Could you check a few things on this model? Use its own coordinates, in mm. Face numbers are marked on the shaded views. A direction names the side the tool comes from. Coordinates: 2 decimals unless noted, no trailing zeros. Loops run counter-clockwise (first coordinate to the right, second up) from the corner with the lowest first, then second, coordinate; pieces in that order, holes last. Notation, with made-up numbers: (45.5, -24.75) -> (79.5, -24.75) arc R17 ccw to (79.5, -3.75) -> close; hole circle Ø4 at (19, -26.75). An arc over 180 degrees is marked (long way). One line per question, with ' | ' between items. Start each with the question number.
(1) Which directions (+Z, -Z, +X, -X, +Y, -Y) give clear straight access to the entire face, cutting with the end or side of a thin tool? Please do the marked faces 4, 5 and 6.
(2) I'm going to push flat-ended pins straight in: pin 1 Ø3 at (x, y) = (63.41, -68.5) entering from -Z; pin 2 Ø8 at (x, y) = (-31, 20.5) entering from -Z; pin 3 Ø6 at (x, z) = (98.5, 6) entering from +Y; pin 4 Ø4 at (y, z) = (-39.5, -7.5) entering from +X. Where does each tip first touch, or does it pass through?
(3) If I drill on line 1 along Z through (x, y) = (46, 53.5); line 2 along X through (y, z) = (-3, 16); line 3 along Z through (x, y) = (-32, -21.5), over which ranges is the centre line in solid material (lowest first)?
(4) Suppose I cut it at A-A (x = -6.5). Please give me the cut outline in (y, z), plus the area to 3 significant figures.
(5) Suppose I cut it at B-B (x = -50). Please give me the cut outline in (y, z).
(6) If we mould it in two halves opening along X, with no side actions, what happens to the marked faces 1, 2 and 3? For each: pulls with the +X half, pulls with the -X half, needs draft (parallel to the pull), parting line crosses it, or undercut.
```python
from build123d import *

# Parameters (mm, degrees)
SKETCH1_4_RX        = 3.738629792
SKETCH1_4_RY        = 2.663157663
SKETCH1_4_R         = 0.723268125
SKETCH1_4_R_2       = 0.681301536
SKETCH1_4_R_3       = 0.980026241
SKETCH1_4_R_4       = 0.97959392
BOSS_EXTRUDE1_DEPTH = 0.254
BOSS_EXTRUDE2_DEPTH = 1.27
CIRPATTERN1_COUNT   = 4
FILLET1_R           = 1.27
SCALE1_SCALE        = 2.276
SKETCH2_R           = 2.38125
CUT_EXTRUDE1_DEPTH  = 50.083123014


with BuildPart() as part:
    # Sketch1 → Revolve1 (revolve)
    with BuildSketch(Plane.XY):
        with BuildLine():
            add(Edge.make_bspline(
                [(77.770736546, 14.197719485), (83.967767677, 14.197719485), (96.645248899, 10.827489794)],
                knots=[0, 0, 0, 1, 1, 1], degree=2))
            Line((96.645248899, 10.827489794), (96.645248899, 0))
            Line((96.645248899, 0), (17.093728294, 0))
            Line((17.093728294, 0), (17.093728294, 18.913287876))
            ThreePointArc((17.093728294, 18.913287876), (17.697865454, 20.511952721), (19.208297022, 21.311519777))
            Line((19.208297022, 21.311519777), (33.085444719, 21.311519777))
            Line((33.085444719, 21.311519777), (34.249634962, 20.65957324))
            Line((34.249634962, 20.65957324), (37.67078875, 20.65957324))
            Line((37.67078875, 20.65957324), (37.67078875, 21.107528589))
            Line((37.67078875, 21.107528589), (59.2694473, 21.107528589))
            Line((59.2694473, 21.107528589), (60.005153989, 20.695532843))
            Line((60.005153989, 20.695532843), (69.857537365, 20.695532843))
            Line((69.857537365, 20.695532843), (74.312442602, 17.349227048))
            Line((74.312442602, 17.349227048), (74.909379663, 17.349227048))
            Line((74.909379663, 17.349227048), (74.981675377, 14.952840317))
            Line((74.981675377, 14.952840317), (77.770736546, 14.952840317))
            Line((77.770736546, 14.952840317), (77.770736546, 14.197719485))
        make_face()
        with BuildLine():
            ThreePointArc((0, 0), (0.275579454, 2.642942048), (1.090462068, 5.172181663))
            Line((1.090462068, 5.172181663), (9.450406563, 5.172181663))
            Line((9.450406563, 5.172181663), (9.450406563, 0))
            Line((9.450406563, 0), (0, 0))
        make_face()
        Polygon((37.67078875, 18.679077388), (37.67078875, 20.65957324), (37.67078875, 21.107528589), (59.2694473, 21.107528589), (59.2694473, 18.679077388), align=None)
    revolve(axis=Axis((-26.796271974, 0, 0), (1, 0, 0)))

    # Sketch1_4 → Boss-Extrude1 (add, symmetric)
    with BuildSketch(Plane.XY):
        with BuildLine():
            ThreePointArc((57.062667076, 33.029408208), (58.562948924, 32.411407764), (59.192673253, 30.916009008))
            Line((59.192673253, 30.916009008), (59.2694473, 21.107528589))
            Line((59.2694473, 21.107528589), (37.67078875, 21.107528589))
            Line((37.67078875, 21.107528589), (37.67078875, 30.916009008))
            ThreePointArc((37.67078875, 30.916009008), (38.289789045, 32.410407913), (39.784187951, 33.029408208))
            Line((39.784187951, 33.029408208), (57.062667076, 33.029408208))
        make_face()
        with Locations((48.297023122, 27.463003731)):
            Ellipse(SKETCH1_4_RX, SKETCH1_4_RY, mode=Mode.SUBTRACT)
        with Locations((54.025364363, 23.762393902)):
            Circle(SKETCH1_4_R, mode=Mode.SUBTRACT)
        with Locations((42.682741772, 23.762393902)):
            Circle(SKETCH1_4_R_2, mode=Mode.SUBTRACT)
        with Locations((40.895803465, 30.126161394)):
            Circle(SKETCH1_4_R_3, mode=Mode.SUBTRACT)
        with Locations((55.916505535, 30.126161394)):
            Circle(SKETCH1_4_R_4, mode=Mode.SUBTRACT)
        Polygon((37.67078875, 18.679077388), (37.67078875, 20.65957324), (37.67078875, 21.107528589), (59.2694473, 21.107528589), (59.2694473, 18.679077388), align=None)
    boss_extrude1 = extrude(amount=BOSS_EXTRUDE1_DEPTH, both=True)

    # Sketch1_5 → Boss-Extrude2 (add, symmetric)
    with BuildSketch(Plane.XY):
        with BuildLine():
            ThreePointArc((11.014724068, 6.119928269), (10.364916389, 5.427600899), (9.450406563, 5.172181663))
            Line((9.450406563, 5.172181663), (9.450406563, 0))
            Line((9.450406563, 0), (12.123394722, 0))
            Line((12.123394722, 0), (12.123394722, 4.941548024))
            Line((12.123394722, 4.941548024), (17.093728294, 14.456770177))
            Line((17.093728294, 14.456770177), (17.093728294, 17.757592992))
            Line((17.093728294, 17.757592992), (11.971268091, 7.951139141))
            Line((11.971268091, 7.951139141), (11.014724068, 6.119928269))
        make_face()
    boss_extrude2 = extrude(amount=BOSS_EXTRUDE2_DEPTH, both=True)

    # Sketch1_6 → Cut-Revolve1 (revolve, cut)
    with BuildSketch(Plane.XY):
        with BuildLine():
            Line((9.450406563, 7.951139141), (9.450406563, 5.172181663))
            ThreePointArc((9.450406563, 5.172181663), (10.364916389, 5.427600899), (11.014724068, 6.119928269))
            Line((11.014724068, 6.119928269), (11.971268091, 7.951139141))
            Line((11.971268091, 7.951139141), (9.450406563, 7.951139141))
        make_face()
    cut_revolve1 = revolve(axis=Axis((-26.796271974, 0, 0), (1, 0, 0)), mode=Mode.SUBTRACT)

    # CirPattern1: Boss-Extrude2, Cut-Revolve1 ×4 about axis
    cirpattern1_axis = Axis((0, 0, 0), (1, 0, 0))
    for i in range(1, CIRPATTERN1_COUNT):
        add(boss_extrude2.rotate(cirpattern1_axis, i * 360 / CIRPATTERN1_COUNT))
        add(cut_revolve1.rotate(cirpattern1_axis, i * 360 / CIRPATTERN1_COUNT), mode=Mode.SUBTRACT)

    # Mirror1: Boss-Extrude1 across plane
    add(boss_extrude1.mirror(Plane.ZX))

    # Fillet1
    fillet1_edges = [part.edges().sort_by_distance(p)[0] for p in [
        (1.090462068, -5.172181663, 0),
    ]]
    fillet(fillet1_edges, radius=FILLET1_R)


with BuildPart() as part_1:
    # Scale1: scaled about (50.004637092, -1.3e-08, 0)
    add(part.part.scale(SCALE1_SCALE).moved(Location((-63.805916929, 1.7e-08, 0))))

    # Sketch2 → Cut-Extrude1 (cut, through all)
    with BuildSketch(Plane.XY.offset(0.578104003)):
        with Locations((29.405893819, 68.5)):
            Circle(SKETCH2_R)
        with Locations((63.405893819, 68.5)):
            Circle(SKETCH2_R)
        with Locations((29.405893819, -68.5)):
            Circle(SKETCH2_R)
        with Locations((63.405893819, -68.5)):
            Circle(SKETCH2_R)
    extrude(amount=-CUT_EXTRUDE1_DEPTH, mode=Mode.SUBTRACT)


solid = part_1.part
```
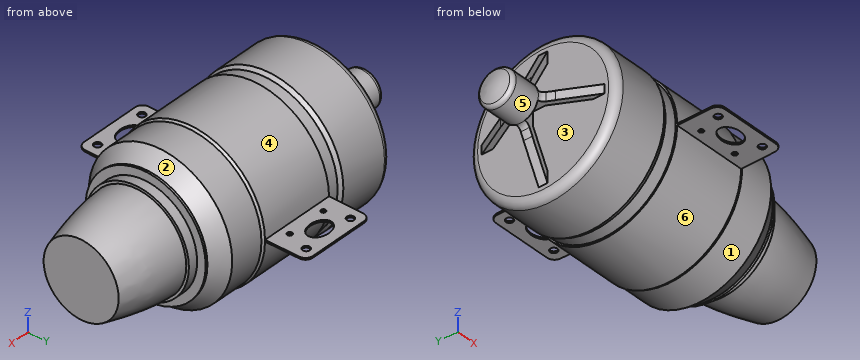
Checks:
1) face 4: +Z, +X | face 5: -X | face 6: -Z, +X
2) pin 1: passes through | pin 2: stops at z = -2.89 | pin 3: stops at y = 46.51 | pin 4: stops at x = 106.73
3) line 1: z = -0.58 to 0.58 | line 2: x = -24.9 to 156.16 | line 3: z = -2.89 to 2.89
4) outline: circle Ø97.01 at (0, 0) | area: 7,390 mm^2
5) outline: circle Ø23.54 at (0, 0)
6) face 1: needs draft | face 2: pulls with the +X half | face 3: undercut
